```python
from build123d import *

# Parameters (mm, degrees)
SKICA1_W                = 300
SKICA1_H                = 300
P_IDAT_VYSUNUT_M1_DEPTH = 10
SKICA3_R                = 40.135302542
SKICA3_R_2              = 32.941200184
P_IDAT_VYSUNUT_M3_DEPTH = 10


with BuildPart() as part:
    # Skica1 → Přidat vysunutím1 (new body)
    with BuildSketch(Plane.XY):
        with Locations((150, 150)):
            Rectangle(SKICA1_W, SKICA1_H)
    extrude(amount=P_IDAT_VYSUNUT_M1_DEPTH)

    # Skica3 → Přidat vysunutím3 (add)
    # profile 1 of 9: a face of its own
    with BuildSketch(Plane.XY.offset(10)):
        with Locations((165.026842843, 104.272964979)):
            Circle(SKICA3_R)
        with Locations((165.026842843, 104.272964979)):
            Circle(SKICA3_R_2, mode=Mode.SUBTRACT)
    # profile 2 of 9: a face of its own
    with BuildSketch(Plane.XY.offset(10)):
        with BuildLine():
            Line((134.114323402, 155.810428325), (135.178982609, 131.104807063))
            ThreePointArc((135.178982609, 131.104807063), (144.916831788, 139.006665697), (156.618002898, 143.517504994))
            Line((156.618002898, 143.517504994), (134.114323402, 155.810428325))
        make_face()
    # profile 3 of 9: a face of its own
    with BuildSketch(Plane.XY.offset(10)):
        with BuildLine():
            ThreePointArc((188.438271645, 182.463164069), (165.555400469, 170.31094498), (165.733072295, 144.402053558))
            ThreePointArc((165.733072295, 144.402053558), (176.734461574, 142.662731504), (186.834212062, 137.966898527))
            ThreePointArc((186.834212062, 137.966898527), (179.680788671, 160.50181988), (188.438271645, 182.463164069))
        make_face()
    # profile 4 of 9: a face of its own
    with BuildSketch(Plane.XY.offset(10)):
        with BuildLine():
            Line((216.564306188, 135.185484421), (191.858684926, 134.120825214))
            ThreePointArc((191.858684926, 134.120825214), (199.76054356, 124.382976034), (204.271382857, 112.681804924))
            Line((204.271382857, 112.681804924), (216.564306188, 135.185484421))
        make_face()
    # profile 5 of 9: a face of its own
    with BuildSketch(Plane.XY.offset(10)):
        with BuildLine():
            ThreePointArc((243.217041932, 80.861536177), (231.064822844, 103.744407353), (205.155931421, 103.566735527))
            ThreePointArc((205.155931421, 103.566735527), (203.416609367, 92.565346248), (198.72077639, 82.46559576))
            ThreePointArc((198.72077639, 82.46559576), (221.255697743, 89.619019151), (243.217041932, 80.861536177))
        make_face()
    # profile 6 of 9: a face of its own
    with BuildSketch(Plane.XY.offset(10)):
        with BuildLine():
            ThreePointArc((194.874703077, 77.441122896), (185.136853898, 69.539264262), (173.435682787, 65.028424965))
            Line((173.435682787, 65.028424965), (195.939362284, 52.735501634))
            Line((195.939362284, 52.735501634), (194.874703077, 77.441122896))
        make_face()
    # profile 7 of 9: a face of its own
    with BuildSketch(Plane.XY.offset(10)):
        with BuildLine():
            ThreePointArc((164.32061339, 64.143876401), (153.319224112, 65.883198455), (143.219473624, 70.579031432))
            ThreePointArc((143.219473624, 70.579031432), (150.372897014, 48.044110079), (141.615414041, 26.08276589))
            ThreePointArc((141.615414041, 26.08276589), (164.498285217, 38.234984979), (164.32061339, 64.143876401))
        make_face()
    # profile 8 of 9: a face of its own
    with BuildSketch(Plane.XY.offset(10)):
        with BuildLine():
            ThreePointArc((138.195000759, 74.425104745), (130.293142125, 84.162953925), (125.782302829, 95.864125035))
            Line((125.782302829, 95.864125035), (113.489379497, 73.360445538))
            Line((113.489379497, 73.360445538), (138.195000759, 74.425104745))
        make_face()
    # profile 9 of 9: a face of its own
    with BuildSketch(Plane.XY.offset(10)):
        with BuildLine():
            ThreePointArc((124.897754265, 104.979194432), (126.637076319, 115.980583711), (131.332909296, 126.080334199))
            ThreePointArc((131.332909296, 126.080334199), (108.797987942, 118.926910808), (86.836643754, 127.684393782))
            ThreePointArc((86.836643754, 127.684393782), (98.988862842, 104.801522606), (124.897754265, 104.979194432))
        make_face()
    extrude(amount=P_IDAT_VYSUNUT_M3_DEPTH)


solid = part.part
```
Here's how the part is built. I have some questions about the finished solid (model axes, mm). A direction names the side the tool comes from. Give positions to 0.01 mm unless a question says otherwise; leave off trailing zeros. Write each loop counter-clockwise with the first axis right and the second up, starting at its lowest first coordinate (ties: lowest second). Pieces come first, ordered by that corner, then holes. Notation, with made-up numbers: M 41.25,41 L 70.25,41 A21 ccw 70.25,68 Z; hole C 8.25,58 d4. An arc over 180 degrees is marked long. Put each result on its own line as item: value. Start each with the question number.
Item 1: On a 3-axis mill with a long thin cutter (end or side, diameter ignored), from which of +Z, -Z, +X, -X, +Y, -Y can I reach the whole of each face in a straight line? I mean faces 5 (the cylindrical face through (220.92, 89.63, 14.93)), 6 (the cylindrical face through (195.456, 91.656, 14.93)), 7 (the cylindrical face through (150.383, 48.382, 14.93)), 8 (the flat face through (195.414, 64.915, 14.93)). Say none if no direction works.
Item 2: If we section it at D-D, the plane y = 159.5: Write out the boundary of the cut face in (x, z), then the cut area to 3 significant figures.
Item 3: If we section it at A-A, the plane z = 15: Write out the boundary of the cut face in (x, y) (1 decimal), then the cut area to 3 significant figures.
Item 4: If we section it at B-B, the plane y = 232: Write out the boundary of the cut face in (x, z).
Item 5: Thinking about a two-plate mould opening in X: for faces 1 (the flat face through (125.669, 73.885, 14.93)), 2 (the flat face through (0, 148, 5)), 3 (the flat face through (148, 152, 0)), 4 (the cylindrical face through (109.135, 118.916, 14.93)), which applies, +X half, -X half, draft (parallel to the pull), parting line (faces both ways), or undercut?
Item 6: I need wall thicknesses on L1, parallel to Z at x = 64, y = 250.5; L2, parallel to X at y = 77.5, z = 14.5; L3, parallel to X at y = 79.5, z = 12.5. Which ranges of each line are inside material? Lowest first, please. Write a range as from..to.
Item 7: Will this pin go through, and if not, where does the flat tip stop? pin 1 (12 mm diameter, centred on y = 168, z = 17.5, fed in from +X).
Values:
1. face 5: +Z, -Y
1. face 6: +Z
1. face 7: +Z, -X
1. face 8: +Z, +X
2. outline: M 0,0 L 300,0 L 300,10 L 179.66,10 L 179.66,20 L 162.11,20 L 162.11,10 L 0,10 Z
2. area: 3,180 mm²
3. outline: M 86.8,127.7 A25 ccw 124.9,105 A40.1 ccw 125.8,95.9 L 113.5,73.4 L 138.2,74.4 A40.1 ccw 143.2,70.6 A35.1 cw 141.6,26.1 A25 ccw 164.3,64.1 A40.1 ccw 173.4,65 L 195.9,52.7 L 194.9,77.4 A40.1 ccw 198.7,82.5 A35.1 cw 243.2,80.9 A25 ccw 205.2,103.6 A40.1 ccw 204.3,112.7 L 216.6,135.2 L 191.9,134.1 A40.1 ccw 186.8,138 A35.1 cw 188.4,182.5 A25 ccw 165.7,144.4 A40.1 ccw 156.6,143.5 L 134.1,155.8 L 135.2,131.1 A40.1 ccw 131.3,126.1 A35.1 cw Z; hole C 165,104.3 d65.9
3. area: 5,140 mm²
4. outline: M 0,0 L 300,0 L 300,10 L 0,10 Z
5. face 1: undercut
5. face 2: -X half
5. face 3: draft
5. face 4: undercut
6. L1: 0..10
6. L2: 115.75..145.83, 184.22..194.93
6. L3: 116.84..143.31, 186.74..196.6
7. pin 1: x = 182.91
